For this review, take the finished solid that the model builds, in its own axes (mm). Face numbers are marked on the shaded views. A direction names the side the tool comes from. Give positions to 0.01 mm unless a question says otherwise; leave off trailing zeros. Loops run counter-clockwise (first coordinate to the right, second up) from the corner with the lowest first, then second, coordinate; pieces in that order, holes last.
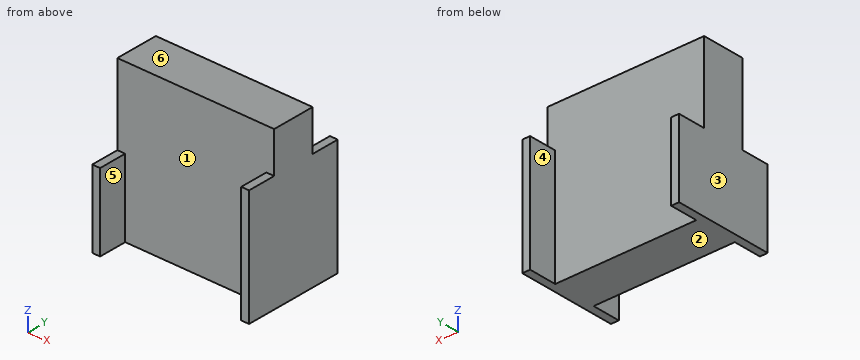
```python
from build123d import *

# Parameters (mm, degrees)
SKETCH1_W           = 50
SKETCH1_H           = 50
BOSS_EXTRUDE1_DEPTH = 15.9
SKETCH2_W           = 45
SKETCH2_H           = 9
CUT_EXTRUDE1_DEPTH  = 59.118929791
SKETCH3_W           = 13
SKETCH3_H           = 9
CUT_EXTRUDE2_DEPTH  = 56.982675892
SKETCH4_W           = 25.5
SKETCH4_H           = 9
CUT_EXTRUDE3_DEPTH  = 56.982675892


with BuildPart() as part:
    # Sketch1 → Boss-Extrude1 (new, symmetric)
    with BuildSketch(Plane(origin=(0, 0, 0), x_dir=(1, 0, 0), z_dir=(0, 1, 0))):
        Rectangle(SKETCH1_W, SKETCH1_H)
    extrude(amount=BOSS_EXTRUDE1_DEPTH, both=True)

    # Sketch2 → Cut-Extrude1 (cut, through all)
    with BuildSketch(Plane.XY.offset(25)):
        with Locations((0, 11.4)):
            Rectangle(SKETCH2_W, SKETCH2_H)
    cut_extrude1 = extrude(amount=-CUT_EXTRUDE1_DEPTH, mode=Mode.SUBTRACT)

    # Sketch3 → Cut-Extrude2 (cut, through all)
    with BuildSketch(Plane.ZY.offset(-22.5)):
        with Locations((18.5, 11.4)):
            Rectangle(SKETCH3_W, SKETCH3_H)
    cut_extrude2 = extrude(amount=-CUT_EXTRUDE2_DEPTH, mode=Mode.SUBTRACT)

    # Sketch4 → Cut-Extrude3 (cut, through all)
    with BuildSketch(Plane(origin=(-22.5, 0, 0), x_dir=(0, 0, -1), z_dir=(1, 0, 0))):
        with Locations((-12.25, 11.4)):
            Rectangle(SKETCH4_W, SKETCH4_H)
    cut_extrude3 = extrude(amount=-CUT_EXTRUDE3_DEPTH, mode=Mode.SUBTRACT)

    # Mirror1: Cut-Extrude1, Cut-Extrude2, Cut-Extrude3 across plane
    add(cut_extrude1.mirror(Plane.ZX), mode=Mode.SUBTRACT)
    add(cut_extrude2.mirror(Plane.ZX), mode=Mode.SUBTRACT)
    add(cut_extrude3.mirror(Plane.ZX), mode=Mode.SUBTRACT)


solid = part.part
```
Q1. Consider section D-D on x = 1. Give the boundary of the cut face in (y, z), plus the area to 3 significant figures.
Answers:
outline: (-6.9, -25) - (6.9, -25) - (6.9, 25) - (-6.9, 25) - close
area: 690 mm2
Q2. Consider section B-B on z = 5. Give the boundary of the cut face in (x, y), plus the area to 3 significant figures.
Answers:
outline: (-25, -6.9) - (22.5, -6.9) - (22.5, -15.9) - (25, -15.9) - (25, 15.9) - (22.5, 15.9) - (22.5, 6.9) - (-25, 6.9) - close
area: 735 mm2
Q3. For pin 1 Ø10 at (x, z) = (-10.5, 2.5) entering from +Y; pin 2 Ø1.5 at (x, y) = (11.5, -7) entering from +Z; pin 3 Ø1.2 at (x, y) = (-24.5, -10.5) entering from +Z; pin 4 Ø3 at (x, y) = (24, 13) entering from +Z, all flat-tipped, find the tip position at first contact; note any pin that passes through.
Answers:
pin 1: stops at y = 6.9
pin 2: stops at z = 25
pin 3: stops at z = -0.5
pin 4: stops at z = 12
Q4. Mouldability with a two-part tool opening along X and no side actions: class the marked faces 1, 2, 3 and 4 as +X half, -X half, draft (parallel to the pull), parting line (faces both ways), or undercut.
Answers:
face 1: undercut
face 2: draft
face 3: -X half
face 4: undercut
Q5. Consider section A-A on y = 12. Give the boundary of the cut face in (x, z), plus the area to 3 significant figures.
Answers:
outline: (-25, -25) - (-22.5, -25) - (-22.5, -0.5) - (-25, -0.5) - close; (22.5, -25) - (25, -25) - (25, 12) - (22.5, 12) - close
area: 154 mm2
Q6. For probe 1 along X at (y, z) = (-13, -19.5); probe 2 along Y at (x, z) = (18.5, -13), list the stretches that pass through material, from the lowest coordinate up.
Answers:
probe 1: x = -25 to -22.5, 22.5 to 25
probe 2: y = -6.9 to 6.9
Q7. Machinability: for the marked faces 5 and 6, which of the approach directions +Z, -Z, +X, -X, +Y, -Y give a long, thin tool a straight path to every point of the face, cutting with its end or side? Answer none if there is none.
Answers:
face 5: +Z, -Z, -Y
face 6: +Z, +X, -X, +Y, -Y
Q8. Consider section C-C on z = -4.5. Give the boundary of the cut face in (x, y), plus the area to 3 significant figures.
Answers:
outline: (-25, -15.9) - (-22.5, -15.9) - (-22.5, -6.9) - (22.5, -6.9) - (22.5, -15.9) - (25, -15.9) - (25, 15.9) - (22.5, 15.9) - (22.5, 6.9) - (-22.5, 6.9) - (-22.5, 15.9) - (-25, 15.9) - close
area: 780 mm2
